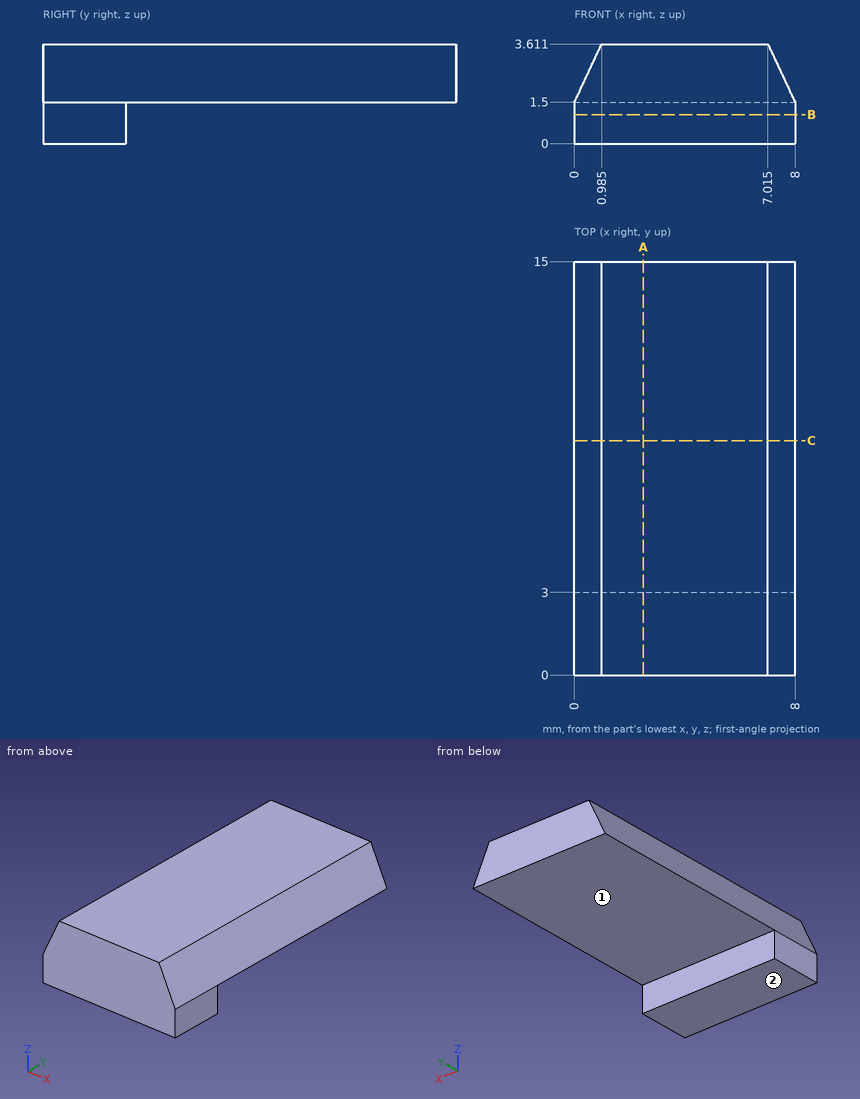
Job drawing, mm, ordinate dimensions from the low corner. One solid piece. A direction names the side the tool comes from. Give positions to 0.01 mm unless a question says otherwise; leave off trailing zeros. Loops run counter-clockwise (first coordinate to the right, second up) from the corner with the lowest first, then second, coordinate; pieces in that order, holes last. Notation, with made-up numbers: (60.5, 86.25) -> (70.5, 86.25) arc R20 cw to (70.5, 98.25) -> close; hole circle Ø10 at (-2.75, -11). An arc over 180 degrees is marked (long way). Write each question's results on one line, items separated by ' | '.
(1) Flat gauge pin, fed straight in: pin 1 Ø4 at (x, y) = (3, 6) entering from -Z. Where does the tip first touch, or does it go through?
Geometry results:
pin 1: stops at z = 1.5
(2) Tool access for the marked faces 1 and 2: list every direction of +Z, -Z, +X, -X, +Y, -Y with a clear straight run to the whole face (end or side of a thin tool).
Geometry results:
face 1: -Z, +X, -X, +Y | face 2: -Z, +X, -X, +Y, -Y
(3) Cut at C-C on y = 8.5. List the corners of the cut face in (x, z) (1 decimal).
Geometry results:
outline: (0, 1.5) -> (8, 1.5) -> (7, 3.6) -> (1, 3.6) -> close
(4) Cut at B-B on z = 1.05. List the corners of the cut face in (x, y), and give its area (3 significant figures).
Geometry results:
outline: (0, 0) -> (8, 0) -> (8, 3) -> (0, 3) -> close | area: 24.0 mm²
(5) Probe line 1 along Z through (x, y) = (3.25, 10.25); line 2 along Y through (x, z) = (6.25, 1.05); line 3 along X through (y, z) = (4, 1.85) (1 decimal). List the from-to ranges inside material, lowest first.
Geometry results:
line 1: z = 1.5 to 3.61 | line 2: y = 0 to 3 | line 3: x = 0.2 to 7.8
(6) Cut at A-A on x = 2.5. List the corners of the cut face in (y, z).
Geometry results:
outline: (0, 0) -> (3, 0) -> (3, 1.5) -> (15, 1.5) -> (15, 3.61) -> (0, 3.61) -> close
